Geometry check sheet. Reference: the model listing, model coordinates, mm. A direction names the side the tool comes from. Round coordinates to 2 decimals unless told otherwise and drop trailing zeros. Order: outer loops, then holes, each group sorted by start corner. A loop starts at its lowest first (then second) coordinate and runs counter-clockwise, first axis right, second up. Notation, with made-up numbers: (57.5, -29.75) - (87.5, -29.75) arc R35 cw to (87.5, 9.25) - close; hole circle Ø8 at (35, 44.25). An arc over 180 degrees is marked (long way). One line per question, with ' | ' between items. Start each with the question number.
Q1. Tool access check on faces 1 (the face through (-6.26, 0.3, 5.06)), 2 (the face through (-17.387, -4.499, 0.198)), 3 (the face through (-17.387, -4.499, 9.802)), 4 (the face through (-2, 9, 0)), 5 (the face through (-8.463, 10.499, 9.802)). Record the directions out of +Z, -Z, +X, -X, +Y, -Y that give a thin tool (end or side, any length) a straight path to the whole face; none if there is none.
Q2. Mould release check, pull along X, two halves, no side actions. Record for faces 6 (the face through (8.69, 10.7, 5.06)), 7 (the face through (-16.59, -0.3, 5.06)), 8 (the face through (-11, 0, 5)), 9 (the face through (-9.12, 3.17, 9.69)): +X half, -X half, draft (parallel to the pull), parting line (faces both ways), or undercut.
Q3. Sectioned sample at A-A, the plane y = -2. Enter the section's corners in (x, z) (3 decimals), then the cut area to 3 significant figures.
Q4. Material ranges on line 1 along X through (y, z) = (1.25, 5.25) (3 decimals); line 2 along X through (y, z) = (7, 1) (3 decimals); line 3 along X through (y, z) = (10, 2.25) (3 decimals), recorded low to high.
Q5. Sectioned sample at B-B, the plane x = 2.5. Enter the section's corners in (y, z), then the cut area to 3 significant figures.
Q6. Sectioned sample at C-C, the plane y = 9.25. Enter the section's corners in (x, z) (3 decimals).
Q7. Gauge pin test, flat ends, axial feed: P1, Ø3, axis at y = 8, z = 6, coming from the -X side (3 decimals); P2, Ø4.5, axis at x = 13, z = 3, coming from the -Y side; P3, Ø4, axis at x = -0.5, z = 2, coming from the -Y side. Record the tip position at first contact, or that the pin passes through.
```python
from build123d import *

# Parameters (mm, degrees)
BOSS_EXTRUDE1_DEPTH = 10
FILLET1_R           = 1
CHAMFER1_SIZE       = 0.5


with BuildPart() as part:
    # Sketch1 → Boss-Extrude1 (new body)
    with BuildSketch(Plane.XY):
        Polygon((-5.975, 0), (-5.975, 8), (5.975, 8), (5.975, 0), (16.875, 0), (16.875, -5), (23.125, -5), (23.125, 0), (23.125, 3), (8.975, 3), (8.975, 11), (-8.975, 11), (-8.975, 3), (-23.125, 3), (-23.125, 0), (-23.125, -5), (-16.875, -5), (-16.875, 0), align=None)
    extrude(amount=BOSS_EXTRUDE1_DEPTH)

    # Fillet1
    fillet1_edges = [part.edges().sort_by_distance(p)[0] for p in [
        (-16.875, 0, 5),
        (-16.875, -5, 5),
        (-23.125, -5, 5),
        (-23.125, 3, 5),
        (-8.975, 3, 5),
        (-8.975, 11, 5),
        (8.975, 11, 5),
        (23.125, 3, 5),
        (23.125, -5, 5),
        (16.875, -5, 5),
        (16.875, 0, 5),
        (5.975, 0, 5),
        (5.975, 8, 5),
        (-5.975, 8, 5),
        (-5.975, 0, 5),
    ]]
    fillet(fillet1_edges, radius=FILLET1_R)

    # Chamfer1
    chamfer1_edges = [part.edges().sort_by_distance(p)[0] for p in [
        (16.582106781, -0.292893219, 0),
        (16.582106781, -0.292893219, 10),
        (-5.682106781, 7.707106781, 0),
        (-5.682106781, 7.707106781, 10),
        (5.682106781, 7.707106781, 0),
        (5.682106781, 7.707106781, 10),
        (-9.267893219, 3.292893219, 0),
        (-9.267893219, 3.292893219, 10),
        (-16.582106781, -0.292893219, 0),
        (-16.582106781, -0.292893219, 10),
        (8.975, 6.5, 0),
        (8.975, 6.5, 10),
        (15.55, 3, 0),
        (15.55, 3, 10),
        (-11.425, 0, 0),
        (-16.875, -2.5, 0),
        (-20, -5, 0),
        (-23.125, -1, 0),
        (-16.05, 3, 0),
        (-8.975, 7, 0),
        (0, 11, 0),
        (23.125, -1, 0),
        (20, -5, 0),
        (16.875, -2.5, 0),
        (11.425, 0, 0),
        (5.975, 4, 0),
        (0, 8, 0),
        (-5.975, 4, 0),
        (-22.832106781, -4.707106781, 0),
        (-17.167893219, -4.707106781, 0),
        (-22.832106781, 2.707106781, 0),
        (-8.682106781, 10.707106781, 0),
        (8.682106781, 10.707106781, 0),
        (-6.267893219, 0.292893219, 0),
        (6.267893219, 0.292893219, 0),
        (17.167893219, -4.707106781, 0),
        (22.832106781, -4.707106781, 0),
        (22.832106781, 2.707106781, 0),
        (23.125, -1, 10),
        (-11.425, 0, 10),
        (-5.975, 4, 10),
        (0, 8, 10),
        (5.975, 4, 10),
        (11.425, 0, 10),
        (16.875, -2.5, 10),
        (20, -5, 10),
        (0, 11, 10),
        (-8.975, 7, 10),
        (-16.05, 3, 10),
        (-23.125, -1, 10),
        (-20, -5, 10),
        (-16.875, -2.5, 10),
        (-22.832106781, -4.707106781, 10),
        (-17.167893219, -4.707106781, 10),
        (-22.832106781, 2.707106781, 10),
        (-8.682106781, 10.707106781, 10),
        (8.682106781, 10.707106781, 10),
        (-6.267893219, 0.292893219, 10),
        (6.267893219, 0.292893219, 10),
        (17.167893219, -4.707106781, 10),
        (22.832106781, -4.707106781, 10),
        (22.832106781, 2.707106781, 10),
    ]]
    chamfer(chamfer1_edges, length=CHAMFER1_SIZE)


solid = part.part
```
Determined:
1) face 1: +Z, -Z, -Y | face 2: -Z, -Y | face 3: +Z, -Y | face 4: -Z, +X, -X, +Y, -Y | face 5: +Z, -X, +Y
2) face 6: +X half | face 7: undercut | face 8: undercut | face 9: -X half
3) outline: (-23.125, 0.5) - (-22.625, 0) - (-17.375, 0) - (-16.875, 0.5) - (-16.875, 9.5) - (-17.375, 10) - (-22.625, 10) - (-23.125, 9.5) - close; (16.875, 0.5) - (17.375, 0) - (22.625, 0) - (23.125, 0.5) - (23.125, 9.5) - (22.625, 10) - (17.375, 10) - (16.875, 9.5) - close | area: 124 mm2
4) line 1: x = -23.125 to -5.975, 5.975 to 23.125 | line 2: x = -8.975 to -5.975, 5.975 to 8.975 | line 3: x = -8.975 to 8.975
5) outline: (8, 0.5) - (8.5, 0) - (10.5, 0) - (11, 0.5) - (11, 9.5) - (10.5, 10) - (8.5, 10) - (8, 9.5) - close | area: 29.5 mm2
6) outline: (-8.975, 0.5) - (-8.475, 0) - (8.475, 0) - (8.975, 0.5) - (8.975, 9.5) - (8.475, 10) - (-8.475, 10) - (-8.975, 9.5) - close
7) P1: stops at x = -8.975 | P2: stops at y = 0 | P3: stops at y = 8
